Source: CAD feature listing. Evaluate the final solid. Frame: model axes, mm. A direction names the side the tool comes from. Round coordinates to 2 decimals unless told otherwise and drop trailing zeros. Loops run counter-clockwise (first coordinate to the right, second up) from the corner with the lowest first, then second, coordinate; pieces in that order, holes last. Notation, with made-up numbers: (32, 71.5) -> (48, 71.5) arc R29 cw to (48, 98.5) -> close; hole circle Ø6 at (5, -1.5). An arc over 180 degrees is marked (long way). Put each result on its own line as item: value. Start each with the question number.
1. Contact query for flat-ended pins moving along their axis: pin 1 (2 mm diameter, centred on y = 0.5, z = 6.5, fed in from +X); pin 2 (6 mm diameter, centred on x = -0.5, z = 0.5, fed in from -Y). Output: stop coordinate, or through.
2. Material intervals for L1, parallel to Y at x = 0, z = 0.75; L2, parallel to X at y = -1.5, z = -4.25, sorted ascending.
3. Draft query along X for faces 1 (the cylindrical face through (7.75, -1.72, -7.14)), 2 (the flat face through (3, 3, 7.938)), 3 (the cylindrical face through (1.95, -2.54, -0.21)). Return one class per face: pulls with the +X half, pulls with the -X half, needs draft (parallel to the pull), parting line crosses it, or undercut.
4. Cut plane B-B (z = 5.5). Return the cut outline in (x, y).
5. Set-up query: faces 4 (the cylindrical face through (-1.9, 6.1, 0.8)), 5 (the flat face through (2, -3, -7.938)). Return all of +Z, -Z, +X, -X, +Y, -Y with unobstructed straight access to the full face (end or side cutting, diameter ignored); none if empty.
6. Cut plane A-A (y = 0). Return the cut outline in (x, z).
```python
from build123d import *

# Parameters (mm, degrees)
CHAMFER1_SIZE = 0.1984375
FILLET1_R     = 0.1984375
FILLET2_R     = 0.09921875


with BuildPart() as part:
    # Sketch3 → Revolve1 (revolve)
    with BuildSketch(Plane(origin=(0, 0, 0), x_dir=(0, 0, -1), z_dir=(1, 0, 0))):
        Polygon((7.9375, 7.9375), (6.35, 7.9375), (6.35, 6.3881), (-7.9375, 6.3881), (-7.9375, 3.2004), (7.9375, 3.2004), align=None)
    revolve(axis=Axis((0, 0, -7.9375), (0, 0, 1)))

    # Chamfer1
    chamfer1_edges = [part.edges().sort_by_distance(p)[0] for p in [
        (0, -3.2004, 7.9375),
        (0, -6.3881, 7.9375),
        (0, -7.9375, -6.35),
    ]]
    chamfer(chamfer1_edges, length=CHAMFER1_SIZE)

    # Fillet1
    fillet1_edges = [part.edges().sort_by_distance(p)[0] for p in [
        (0, -7.9375, -7.9375),
    ]]
    fillet(fillet1_edges, radius=FILLET1_R)

    # Fillet2
    fillet2_edges = [part.edges().sort_by_distance(p)[0] for p in [
        (0, -6.3881, -6.35),
    ]]
    fillet(fillet2_edges, radius=FILLET2_R)


solid = part.part
```
Solution:
1. pin 1: stops at x = 6.39
1. pin 2: stops at y = -6.39
2. L1: y = -6.39 to -3.2, 3.2 to 6.39
2. L2: x = -6.21 to -2.83, 2.83 to 6.21
3. face 1: parting line crosses it
3. face 2: needs draft
3. face 3: undercut
4. outline: circle Ø12.78 at (0, 0); hole circle Ø6.4 at (0, 0)
5. face 4: +Z
5. face 5: -Z, +X, -X, +Y, -Y
6. outline: (-7.94, -7.74) arc R0.2 ccw to (-7.74, -7.94) -> (-3.2, -7.94) -> (-3.2, 7.74) -> (-3.4, 7.94) -> (-6.19, 7.94) -> (-6.39, 7.74) -> (-6.39, -6.25) arc R0.1 cw to (-6.49, -6.35) -> (-7.74, -6.35) -> (-7.94, -6.55) -> close; (3.2, -7.94) -> (7.74, -7.94) arc R0.2 ccw to (7.94, -7.74) -> (7.94, -6.55) -> (7.74, -6.35) -> (6.49, -6.35) arc R0.1 cw to (6.39, -6.25) -> (6.39, 7.74) -> (6.19, 7.94) -> (3.4, 7.94) -> (3.2, 7.74) -> close
